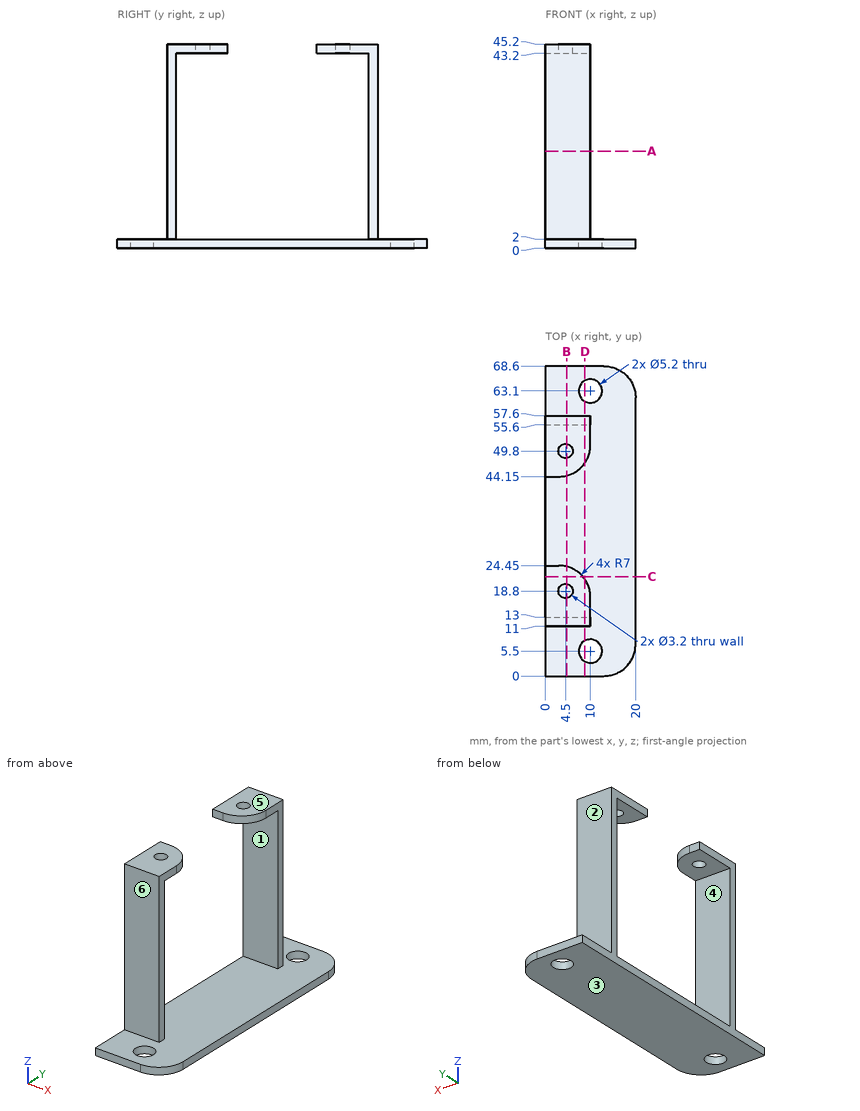
Geometry check sheet. Reference: drawing and pictorial views, mm from the part's lowest x, y, z. A direction names the side the tool comes from. Give positions to 0.01 mm unless a question says otherwise; leave off trailing zeros. Order: outer loops, then holes, each group sorted by start corner. A loop starts at its lowest first (then second) coordinate and runs counter-clockwise, first axis right, second up. Notation, with made-up numbers: M -19.5,78 L 3.5,78 A31 ccw 3.5,117 Z; hole C 43,-12.5 d5. An arc over 180 degrees is marked long. Answer in a Markdown table with one row per item. Add a question column.
Q1. Access from +Z, -Z, +X, -X, +Y, -Y to the whole of each face (thin tool, end or side, straight path). Record for the marked faces 5 and 6.
Q2. Sectioned sample at D-D, the plane x = 8.75. Record the boundary of the cut face in (y, z), and give its area (3 significant figures).
Q3. Sectioned sample at A-A, the plane z = 21.5. Record the boundary of the cut face in (x, y), and give its area (3 significant figures).
Q4. Release check for a two-part mould opening along Z. For the marked faces 1, 2, 3 and 4 record: released by +Z, released by -Z, zero draft, split by the parting line, or undercut.
Q5. Sectioned sample at B-B, the plane x = 4.75. Record the boundary of the cut face in (y, z).
Q6. Gauge pin test, flat ends, axial feed: pin 1 Ø3 at (x, y) = (10, 63.1) entering from -Z; pin 2 Ø8 at (x, z) = (6.5, 19.5) entering from +Y; pin 3 Ø8 at (x, z) = (6.5, 18.5) entering from -Y; pin 4 Ø2.5 at (x, y) = (4.5, 49.8) entering from +Z. Record the tip position at first contact, or that the pin passes through.
Q7. Thickness scan on L1, parallel to Y at x = 10, z = 0.5; L2, parallel to Y at x = 5, z = 34.5; L3, parallel to Y at x = 4.5, z = 43.75. Record the ranges inside material, lowest first.
Q8. Sectioned sample at C-C, the plane y = 22. Record the boundary of the cut face in (x, z), and give its area (3 significant figures).
Verdict:
| question | item | result |
|---|---|---|
| 1 | face 5 | +Z, +X, -X, +Y, -Y |
| 1 | face 6 | +Z, +X, -X, -Y |
| 2 | outline | M 0,0 L 3.22,0 L 3.22,2 L 0,2 Z; M 7.78,0 L 60.82,0 L 60.82,2 L 57.6,2 L 57.6,45.2 L 47.16,45.2 L 47.16,43.2 L 55.6,43.2 L 55.6,2 L 13,2 L 13,43.2 L 21.44,43.2 L 21.44,45.2 L 11,45.2 L 11,2 L 7.78,2 Z; M 65.38,0 L 68.6,0 L 68.6,2 L 65.38,2 Z |
| 2 | area | 326 mm² |
| 3 | outline | M 0,11 L 10,11 L 10,13 L 0,13 Z; M 0,55.6 L 10,55.6 L 10,57.6 L 0,57.6 Z |
| 3 | area | 40.0 mm² |
| 4 | face 1 | undercut |
| 4 | face 2 | zero draft |
| 4 | face 3 | released by -Z |
| 4 | face 4 | undercut |
| 5 | outline | M 0,0 L 68.6,0 L 68.6,2 L 57.6,2 L 57.6,45.2 L 51.38,45.2 L 51.38,43.2 L 55.6,43.2 L 55.6,2 L 13,2 L 13,43.2 L 17.22,43.2 L 17.22,45.2 L 11,45.2 L 11,2 L 0,2 Z; M 20.38,43.2 L 24.23,43.2 L 24.23,45.2 L 20.38,45.2 Z; M 44.37,43.2 L 48.22,43.2 L 48.22,45.2 L 44.37,45.2 Z |
| 6 | pin 1 | through |
| 6 | pin 2 | y = 57.6 |
| 6 | pin 3 | y = 11 |
| 6 | pin 4 | z = 2 |
| 7 | L1 | 0 to 2.9, 8.1 to 60.5, 65.7 to 68.6 |
| 7 | L2 | 11 to 13, 55.6 to 57.6 |
| 7 | L3 | 11 to 17.2, 20.4 to 24.29, 44.31 to 48.2, 51.4 to 57.6 |
| 8 | outline | M 0,0 L 20,0 L 20,2 L 0,2 Z; M 0,43.2 L 8.32,43.2 L 8.32,45.2 L 0,45.2 Z |
| 8 | area | 56.6 mm² |
